Autodesk Inventor part; units mm, degrees
ref_plane "YZ Plane" through (0, 0, 0) normal (1, 0, 0) x (0, 1, 0)
ref_plane "XZ Plane" through (0, 0, 0) normal (0, 1, 0) x (-1, 0, 0)
ref_plane "XY Plane" through (0, 0, 0) normal (0, 0, 1) x (1, 0, 0)
sketch "Sketch1" plane through (0, 0, 0) normal (0, 0, 1) x (1, 0, 0)
  circle A0 centre (0, 0) radius 3
  dimension "d0" = 6
extrude "Extrusion1" add sketch "Sketch1" along normal mid plane 44.5
sketch "Sketch2" plane through (0, 0, 22.25) normal (0, 0, 1) x (1, 0, 0)
  point P0 (0, 0)
  point P1 (0, 0)
hole "Hole1" at (0, 0, 22.25) direction (0, 0, -1) diameter 2.459 depth 8.8 tip angle 118
sketch "Sketch3" plane through (0, 0, 0) normal (0, 1, 0) x (-1, 0, 0)
  line L0 (3, 7.25) -> (2.5, 7.25)
  line L1 (2.5, 7.25) -> (2.5, 12.25)
  line L2 (2.5, 12.25) -> (3, 12.25)
  line L3 (3, 12.25) -> (3, 7.25)
  line L4 (-3, 12.25) -> (-2.5, 12.25)
  line L5 (-2.5, 12.25) -> (-2.5, 7.25)
  line L6 (-2.5, 7.25) -> (-3, 7.25)
  line L7 (-3, 7.25) -> (-3, 12.25)
  line L8 (-3, -22.25) -> (3, -22.25)
  line L9 (3, 22.25) -> (-3, 22.25)
  point P0 (0, 0)
  point P1 (-3, 23.75)
  dimension "d16" = 0.5
  dimension "d17" = 0.5
  dimension "d18" = 5
  dimension "d19" = 10
extrude "Extrusion2" cut sketch "Sketch3" along normal through all both and the other way through all
mirror "Mirror1" about plane through (0, 0, 0) normal (0, 0, 1) of "Hole1"
equation "\"d17\" = d16"
properties part number "Pancake_Lever Weight" material "Aluminum 6061"
Geometry: final body of the model. Coordinates: model frame, mm. A direction names the side the tool comes from. Coordinates: 2 decimals unless noted, no trailing zeros. Order: outer loops, then holes, each group sorted by start corner. A loop starts at its lowest first (then second) coordinate and runs counter-clockwise, first axis right, second up. Notation, with made-up numbers: M 50,33 L 77,33 A25 ccw 77,55 Z; hole C 56,60 d3. An arc over 180 degrees is marked long. Answer in a Markdown table with one row per item. Add a question column.
Q1. Contact query for flat-ended pins moving along their axis: P1, Ø3, axis at y = -2, z = 2.5, coming from the -X side; P2, Ø1.5, axis at x = 0, y = 0, coming from the +Z side; P3, Ø1.5, axis at x = -1.5, z = 7.5, coming from the +Y side. Output: stop coordinate, or through.
Q2. Line query: L1, parallel to Y at x = 0, z = 20; L2, parallel to Y at x = -1, z = -14. Output: solid intervals per line, ascending.
Q3. Section query B-B on y = -2.55. Return the cut outline in (x, z).
Q4. Section query C-C on x = -2. Return the cut outline in (y, z), and give its area (3 significant figures).
Q5. Reachability of faces 1 (the cylindrical face through (-0.748, 0.976, -17.788)), 2 (the flat face through (2.5, 0, 10)), 3 (the cylindrical face through (0.748, 0.976, 17.788)) from +Z, -Z, +X, -X, +Y, -Y: full face, straight path, thin tool, end or side. Return the list, or none.
Q6. Mould query, pull axis X, two halves, no side actions, for faces 4 (the flat face through (1, -1, 22.25)), 5 (the conical face through (0.064, -0.204, 12.84)), 6 (the flat face through (-2.5, 0, 10)). Classes: released by +X, released by -X, zero draft, split by the parting line, or undercut.
Q7. Section query A-A on z = -2. Return the cut outline in (x, y), and give its area (3 significant figures).
Completed:
| question | item | result |
|---|---|---|
| 1 | P1 | stops at x = -2.96 |
| 1 | P2 | stops at z = 13.16 |
| 1 | P3 | stops at y = 2.9 |
| 2 | L1 | y = -3 to -1.23, 1.23 to 3 |
| 2 | L2 | y = -2.83 to -0.72, 0.72 to 2.83 |
| 3 | outline | M -1.58,-22.25 L 1.58,-22.25 L 1.58,22.25 L -1.58,22.25 Z |
| 4 | outline | M -2.24,-22.25 L 2.24,-22.25 L 2.24,22.25 L -2.24,22.25 Z |
| 4 | area | 199 mm2 |
| 5 | face 1 | -Z |
| 5 | face 2 | +X, +Y, -Y |
| 5 | face 3 | +Z |
| 6 | face 4 | zero draft |
| 6 | face 5 | undercut |
| 6 | face 6 | released by -X |
| 7 | outline | C 0,0 d6 |
| 7 | area | 28.3 mm2 |
